```python
from build123d import *

# Parameters (mm, degrees)
F0_W     = 57
F0_H     = 10.75
F1_DEPTH = 11.5
F2_W     = 11.1
F2_H     = 10.75
F3_DEPTH = 10
F4_R     = 1


with BuildPart() as f1:
    # F0 (on Front) → F1 (new body)
    with BuildSketch(Plane.XZ):
        with Locations((0, 0.0343695283)):
            Rectangle(F0_W, F0_H)
    extrude(amount=F1_DEPTH)

    # F2 (on face) → F3 (join)
    with BuildSketch(Plane.XZ.offset(11.5)):
        with Locations((0, 0.0343695283)):
            Rectangle(F2_W, F2_H)
    extrude(amount=F3_DEPTH)

    # F4
    f4_edges = [f1.edges().sort_by_distance(p)[0] for p in [
        (5.55, -21.5, 0.03437),
        (0, -21.5, 5.40937),
        (-5.55, -21.5, 0.03437),
        (0, -21.5, -5.34063),
        (28.5, -11.5, 0.03437),
        (28.5, -5.75, 5.40937),
        (28.5, -5.75, -5.34063),
        (28.5, 0, 0.03437),
        (-28.5, -5.75, 5.40937),
        (-28.5, -11.5, 0.03437),
        (-28.5, -5.75, -5.34063),
        (-28.5, 0, 0.03437),
    ]]
    fillet(f4_edges, radius=F4_R)


solid = f1.part
```
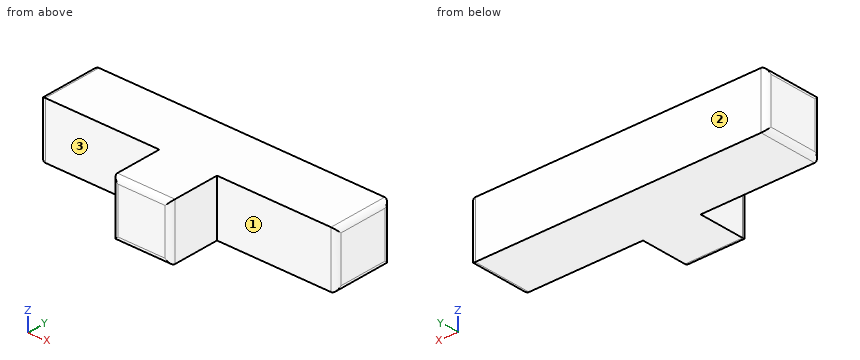
Read the model definition and answer for the solid it produces. Units are mm, in the model's axes. Face numbers are marked on the shaded views. A direction names the side the tool comes from. Give positions to 0.01 mm unless a question says otherwise; leave off trailing zeros. Loops run counter-clockwise (first coordinate to the right, second up) from the corner with the lowest first, then second, coordinate; pieces in that order, holes last.
Item 1: For the marked faces 1, 2 and 3, determine the directions among +Z, -Z, +X, -X, +Y, -Y from which every point of the face is accessible in a straight line to the end or side of a thin tool.
Item 2: The part is cut by section A-A (z = 2.25). Write down the section's boundary in (x, y).
Item 3: The part is cut by section C-C (y = -14.25). Write down the section's boundary in (x, z).
Item 4: The part is cut by section B-B (x = 13). Write down the section's boundary in (y, z), and give its area (3 significant figures).
Item 5: Find the intervals of material crossed by line 1 along X through (y, z) = (-14.5, -1); line 2 along Y through (x, z) = (-6, 4.5); line 3 along X through (y, z) = (-11, 1), in increasing order.
Item 6: Each of these flat-tipped pins is pushed along its axis until it touches: pin 1 Ø4.5 at (y, z) = (-16, -1) entering from -X; pin 2 Ø3 at (x, z) = (16, -1.5) entering from -Y. Where does it stop, or does it pass through?
Taken from the geometry:
1. face 1: +Z, -Z, +X, -Y
1. face 2: +Z, -Z, +X, -X, +Y
1. face 3: +Z, -Z, -X, -Y
2. outline: (-28.5, -10.5) arc R1 ccw to (-27.5, -11.5) - (-5.55, -11.5) - (-5.55, -20.5) arc R1 ccw to (-4.55, -21.5) - (4.55, -21.5) arc R1 ccw to (5.55, -20.5) - (5.55, -11.5) - (27.5, -11.5) arc R1 ccw to (28.5, -10.5) - (28.5, -1) arc R1 ccw to (27.5, 0) - (-27.5, 0) arc R1 ccw to (-28.5, -1) - close
3. outline: (-5.55, -5.34) - (5.55, -5.34) - (5.55, 5.41) - (-5.55, 5.41) - close
4. outline: (-11.5, -5.34) - (0, -5.34) - (0, 5.41) - (-11.5, 5.41) - close
4. area: 124 mm2
5. line 1: x = -5.55 to 5.55
5. line 2: y = -11.5 to 0
5. line 3: x = -28.37 to 28.37
6. pin 1: stops at x = -5.55
6. pin 2: stops at y = -11.5
